from build123d import *

# Parameters (mm, degrees)
SKETCH1_W                       = 104.775
SKETCH1_H                       = 76.2
BOSS_EXTRUDE1_DEPTH             = 187.325
CUT_EXTRUDE1_REACH              = 106.775
SKETCH3_W                       = 101.473
SKETCH3_H                       = 162.56
CUT_EXTRUDE2_DEPTH              = 4.318
SKETCH4_W                       = 89.535
SKETCH4_H                       = 175.133
CUT_EXTRUDE3_DEPTH              = 66.548
CUT_EXTRUDE3_DIRECTION_2_REACH  = 6.318
SKETCH5_W                       = 89.535
SKETCH5_H                       = 15.113
CUT_EXTRUDE4_DEPTH              = 38.1
CUT_EXTRUDE5_DEPTH              = 105.775
SKETCH7_W                       = 5.842
SKETCH7_H                       = 43.18
CUT_EXTRUDE6_DEPTH              = 5.715
CUT_EXTRUDE7_DEPTH              = 22.225
BOSS_EXTRUDE2_REACH             = 54.388
BOSS_EXTRUDE2_DIRECTION_2_REACH = 54.387
CUT_EXTRUDE8_DEPTH              = 104.775
CUT_EXTRUDE9_DEPTH              = 5.969
SKETCH12_W                      = 86.995
SKETCH12_H                      = 164.98932792
CUT_EXTRUDE10_DEPTH             = 2.921
CUT_EXTRUDE11_DEPTH             = 184.007
FILLET1_R                       = 6.35


with BuildPart() as part:
    # Sketch1 → Boss-Extrude1 (new body)
    with BuildSketch(Plane.XY):
        with Locations((52.3875, 38.1)):
            Rectangle(SKETCH1_W, SKETCH1_H)
    extrude(amount=BOSS_EXTRUDE1_DEPTH)

    # Sketch2 → Cut-Extrude1 (cut, up to next)
    with BuildSketch(Plane(origin=(104.775, 0, 0), x_dir=(0, 0, -1), z_dir=(1, 0, 0)), mode=Mode.PRIVATE) as cut_extrude1_sk1:
        Polygon((0, 0), (-4.318, 0), (-4.318, 73.533), (-1.778, 73.533), (-1.778, 63.119), (0, 63.119), align=None)
    cut_extrude1_tool1 = extrude(cut_extrude1_sk1.sketch, amount=-CUT_EXTRUDE1_REACH, mode=Mode.PRIVATE) & part.part
    add(cut_extrude1_tool1.solids().sort_by_distance((104.775, 34.812119, 2.237647))[0], mode=Mode.SUBTRACT)

    # Sketch3 → Cut-Extrude2 (cut)
    with BuildSketch(Plane(origin=(0, 76.2, 0), x_dir=(1, 0, 0), z_dir=(0, 1, 0))):
        with Locations((52.3875, -88.392)):
            Rectangle(SKETCH3_W, SKETCH3_H)
    extrude(amount=-CUT_EXTRUDE2_DEPTH, mode=Mode.SUBTRACT)

    # Sketch4 → Cut-Extrude3 (cut)
    with BuildSketch(Plane(origin=(0, 71.882, 0), x_dir=(1, 0, 0), z_dir=(0, 1, 0))):
        with Locations((52.3875, -94.6785)):
            Rectangle(SKETCH4_W, SKETCH4_H)
    extrude(amount=-CUT_EXTRUDE3_DEPTH, mode=Mode.SUBTRACT)

    # Sketch4 → Cut-Extrude3 direction 2 (cut, up to next)
    with BuildSketch(Plane(origin=(0, 71.882, 0), x_dir=(1, 0, 0), z_dir=(0, 1, 0)), mode=Mode.PRIVATE) as cut_extrude3_direction_2_sk1:
        with Locations((52.3875, -94.6785)):
            Rectangle(SKETCH4_W, SKETCH4_H)
    cut_extrude3_direction_2_tool1 = extrude(cut_extrude3_direction_2_sk1.sketch, amount=CUT_EXTRUDE3_DIRECTION_2_REACH, mode=Mode.PRIVATE) & part.part
    add(cut_extrude3_direction_2_tool1.solids().sort_by_distance((52.3875, 71.882, 94.6785))[0], mode=Mode.SUBTRACT)

    # Sketch5 → Cut-Extrude4 (cut)
    with BuildSketch(Plane(origin=(0, 76.2, 0), x_dir=(1, 0, 0), z_dir=(0, 1, 0))):
        with Locations((52.3875, -179.7685)):
            Rectangle(SKETCH5_W, SKETCH5_H)
    extrude(amount=-CUT_EXTRUDE4_DEPTH, mode=Mode.SUBTRACT)

    # Sketch6 → Cut-Extrude5 (cut, through all)
    with BuildSketch(Plane.ZY):
        Polygon((187.325, 38.1), (187.325, 76.2), (177.927, 76.2), align=None)
    extrude(amount=-CUT_EXTRUDE5_DEPTH, mode=Mode.SUBTRACT)

    # Sketch7 → Cut-Extrude6 (cut)
    with BuildSketch(Plane(origin=(0, 45.741868113, 185.440005865), x_dir=(1, 0, 0), z_dir=(0, 0.239488471, 0.970899208))):
        with Locations((4.699, 13.719081937)):
            Rectangle(SKETCH7_W, SKETCH7_H)
        with Locations((100.076, 13.719081937)):
            Rectangle(SKETCH7_W, SKETCH7_H)
    extrude(amount=-CUT_EXTRUDE6_DEPTH, mode=Mode.SUBTRACT)

    # Sketch8 → Cut-Extrude7 (cut)
    with BuildSketch(Plane(origin=(0, 38.1, 0), x_dir=(1, 0, 0), z_dir=(0, 1, 0))):
        Polygon((92.837, -184.023), (11.938, -184.023), (11.938, -185.293), (17.399, -185.293), (17.399, -187.325), (87.376, -187.325), (87.376, -185.293), (92.837, -185.293), align=None)
    extrude(amount=-CUT_EXTRUDE7_DEPTH, mode=Mode.SUBTRACT)

    # Boss-Extrude2: up to this face of the body (flat: up to its plane)
    boss_extrude2_end = Plane(part.part.faces().sort_by_distance((97.155, 38.338270724, 93.520892383))[0])
    # Sketch9 → Boss-Extrude2 (add, up to the picked face)
    with BuildSketch(Plane(origin=(52.3875, 0, 0), x_dir=(0, 0, -1), z_dir=(1, 0, 0)), mode=Mode.PRIVATE) as boss_extrude2_sk1:
        Polygon((-156.845, 5.334), (-182.245, 5.334), (-182.245, 27.448933333), align=None)
    boss_extrude2_tool1 = split(extrude(boss_extrude2_sk1.sketch, amount=BOSS_EXTRUDE2_REACH, mode=Mode.PRIVATE), bisect_by=boss_extrude2_end, keep=Keep.BOTH, mode=Mode.PRIVATE)
    add(boss_extrude2_tool1.solids().sort_by_distance((52.3875, 12.705644, 173.778333))[0])

    # Boss-Extrude2 direction 2: up to this face of the body (flat: up to its plane)
    boss_extrude2_direction_2_end = Plane(part.part.faces().sort_by_distance((7.62, 38.338270724, 93.520892383))[0])
    # Sketch9 → Boss-Extrude2 direction 2 (add, up to the picked face)
    with BuildSketch(Plane(origin=(52.3875, 0, 0), x_dir=(0, 0, -1), z_dir=(1, 0, 0)), mode=Mode.PRIVATE) as boss_extrude2_direction_2_sk1:
        Polygon((-156.845, 5.334), (-182.245, 5.334), (-182.245, 27.448933333), align=None)
    boss_extrude2_direction_2_tool1 = split(extrude(boss_extrude2_direction_2_sk1.sketch, amount=-BOSS_EXTRUDE2_DIRECTION_2_REACH, mode=Mode.PRIVATE), bisect_by=boss_extrude2_direction_2_end, keep=Keep.BOTH, mode=Mode.PRIVATE)
    add(boss_extrude2_direction_2_tool1.solids().sort_by_distance((52.3875, 12.705644, 173.778333))[0])

    # Sketch10 → Cut-Extrude8 (cut)
    with BuildSketch(Plane(origin=(104.775, 0, 0), x_dir=(0, 0, -1), z_dir=(1, 0, 0))):
        Polygon((-187.325, 10.795), (-187.325, 0), (-164.465, 0), align=None)
    extrude(amount=-CUT_EXTRUDE8_DEPTH, mode=Mode.SUBTRACT)

    # Sketch11 → Cut-Extrude9 (cut)
    with BuildSketch(Plane.ZY):
        Polygon((110.611802523, 69.215), (4.318, 69.215), (4.318, 6.985), (180.34, 6.985), (180.34, 37.251236671), (172.455605046, 69.215), align=None)
    cut_extrude9 = extrude(amount=-CUT_EXTRUDE9_DEPTH, mode=Mode.SUBTRACT)

    # Mirror1: Cut-Extrude9 across plane
    add(cut_extrude9.mirror(Plane(origin=(52.3875, 0, 0), x_dir=(0, 0, 1), z_dir=(1, 0, 0))), mode=Mode.SUBTRACT)

    # Sketch12 → Cut-Extrude10 (cut)
    with BuildSketch(Plane.XZ):
        with Locations((52.3875, 86.81266396)):
            Rectangle(SKETCH12_W, SKETCH12_H)
    extrude(amount=-CUT_EXTRUDE10_DEPTH, mode=Mode.SUBTRACT)

    # Sketch13 → Cut-Extrude11 (cut, through all)
    with BuildSketch(Plane(origin=(0, 0, 4.318), x_dir=(-1, 0, 0), z_dir=(0, 0, -1))):
        Polygon((-5.969, 6.985), (0, 6.985), (0, 1.778), align=None)
        Polygon((-98.806, 6.985), (-104.775, 6.985), (-104.775, 1.778), align=None)
    extrude(amount=-CUT_EXTRUDE11_DEPTH, mode=Mode.SUBTRACT)

    # Fillet1
    fillet1_edges = [part.edges().sort_by_distance(p)[0] for p in [
        (52.3875, 5.334, 7.112),
        (52.3875, 5.334, 156.845),
    ]]
    fillet(fillet1_edges, radius=FILLET1_R)


solid = part.part
Check sheet for the modelled part. Datum: model origin and axes. Units: mm. A direction names the side the tool comes from. Round coordinates to 2 decimals unless told otherwise and drop trailing zeros. Loops run counter-clockwise (first coordinate to the right, second up) from the corner with the lowest first, then second, coordinate; pieces in that order, holes last.
1. Mould release check, pull along Z, two halves, no side actions. Record for faces 6 (the flat face through (3, 22, 180.34)), 7 (the flat face through (52, 5.334, 83)), 8 (the flat face through (101.832, 4.345, 90.563)): released by +Z, released by -Z, zero draft, split by the parting line, or undercut.
2. Sectioned sample at C-C on y = 60.5. Record the boundary of the cut face in (x, z) (3 decimals), and give its area (3 significant figures).
3. Scan lines: probe 1 along Z at (x, y) = (90, 35.5) (3 decimals); probe 2 along X at (y, z) = (24, 27) (3 decimals); probe 3 along X at (y, z) = (71.5, 129) (3 decimals). Record each from-to range of solid material in increasing order.
4. Set-up check for faces 1 (the flat face through (102, 22, 180.34)), 2 (the flat face through (100, 0, 83)), 3 (the cylindrical face through (51.761, 5.748, 156.724)), 4 (the flat face through (51.8, 38.1, 183.6)), 5 (the flat face through (104.775, 72, 114)): record each of +Z, -Z, +X, -X, +Y, -Y from which the full face is reachable in a straight line by a thin tool's end or side.
5. Gauge pin test, flat ends, axial feed: pin 1 Ø3 at (x, z) = (11, 46) entering from +Y; pin 2 Ø5.5 at (x, y) = (43, 35.5) entering from -Z; pin 3 Ø5 at (x, z) = (79, 114.5) entering from -Y. Record the tip position at first contact, or that the pin passes through.
6. Sectioned sample at D-D on x = 15.5. Record the boundary of the cut face in (y, z) (3 decimals).
7. Sectioned sample at A-A on x = 43.5. Record the boundary of the cut face in (y, z) (3 decimals).
8. Sectioned sample at B-B on z = 97.5. Record the boundary of the cut face in (x, y) (3 decimals), and give its area (3 significant figures).
Recorded:
1. face 6: released by -Z
1. face 7: undercut
1. face 8: zero draft
2. outline: (0, 174.605) - (5.969, 174.605) - (5.969, 4.318) - (98.806, 4.318) - (98.806, 174.605) - (104.775, 174.605) - (104.775, 181.8) - (102.997, 181.8) - (102.997, 175.913) - (97.155, 175.913) - (97.155, 7.112) - (7.62, 7.112) - (7.62, 175.913) - (1.778, 175.913) - (1.778, 181.8) - (0, 181.8) - close
2. area: 853 mm2
3. probe 1: z = 4.318 to 7.112, 182.245 to 184.023, 185.293 to 187.325
3. probe 2: x = 5.969 to 7.62, 97.155 to 98.806
3. probe 3: x = 0 to 7.62, 97.155 to 104.775
4. face 1: -Z, +X, -Y
4. face 2: +Z, -Z, +X, -X, -Y
4. face 3: +Y
4. face 4: +Z, +Y
4. face 5: +Z, -Z, +X, +Y, -Y
5. pin 1: stops at y = 5.33
5. pin 2: stops at z = 4.32
5. pin 3: stops at y = 2.92
6. outline: (2.287, 169.307) - (2.921, 169.307) - (2.921, 4.318) - (73.533, 4.318) - (73.533, 1.778) - (63.119, 1.778) - (63.119, 0) - (76.2, 0) - (76.2, 7.112) - (11.684, 7.112) arc R6.35 cw to (5.334, 13.462) - (5.334, 154.468) arc R6.35 cw to (6.895, 158.638) - (27.449, 182.245) - (38.1, 182.245) - (38.1, 184.023) - (15.875, 184.023) - (15.875, 185.293) - (38.1, 185.293) - (38.1, 187.325) - (10.795, 187.325) - close
7. outline: (2.287, 169.307) - (2.921, 169.307) - (2.921, 4.318) - (73.533, 4.318) - (73.533, 1.778) - (63.119, 1.778) - (63.119, 0) - (76.2, 0) - (76.2, 7.112) - (11.684, 7.112) arc R6.35 cw to (5.334, 13.462) - (5.334, 154.468) arc R6.35 cw to (6.895, 158.638) - (27.449, 182.245) - (38.1, 182.245) - (38.1, 184.023) - (15.875, 184.023) - (15.875, 187.325) - (10.795, 187.325) - close
8. outline: (0, 0) - (8.89, 0) - (8.89, 2.921) - (95.885, 2.921) - (95.885, 0) - (104.775, 0) - (104.775, 1.778) - (98.806, 6.985) - (98.806, 69.215) - (104.775, 69.215) - (104.775, 76.2) - (103.124, 76.2) - (103.124, 71.882) - (97.155, 71.882) - (97.155, 5.334) - (7.62, 5.334) - (7.62, 71.882) - (1.651, 71.882) - (1.651, 76.2) - (0, 76.2) - (0, 69.215) - (5.969, 69.215) - (5.969, 6.985) - (0, 1.778) - close
8. area: 559 mm2
